from build123d import *

# Parameters (mm, degrees)
F0_W     = 70
F0_H     = 48
F0_R     = 1.6
F0_H_2   = 10
F1_DEPTH = 3.5
F2_R     = 5
F3_R     = 1


with BuildPart() as f1:
    # F0 (on Front) → F1 (new body)
    with BuildSketch(Plane.XZ):
        with Locations((18, 29)):
            Rectangle(F0_W, F0_H)
        with Locations((-11.999999, 12)):
            Circle(F0_R, mode=Mode.SUBTRACT)
        with Locations((0, 12)):
            Circle(F0_R, mode=Mode.SUBTRACT)
        with Locations((12, 12)):
            Circle(F0_R, mode=Mode.SUBTRACT)
        with Locations((24.000001, 12)):
            Circle(F0_R, mode=Mode.SUBTRACT)
        with Locations((36, 12)):
            Circle(F0_R, mode=Mode.SUBTRACT)
        with Locations((48, 12)):
            Circle(F0_R, mode=Mode.SUBTRACT)
        with Locations((-11.999999, 24)):
            Circle(F0_R, mode=Mode.SUBTRACT)
        with Locations((0, 24)):
            Circle(F0_R, mode=Mode.SUBTRACT)
        with Locations((-11.999999, 36)):
            Circle(F0_R, mode=Mode.SUBTRACT)
        with Locations((0, 36)):
            Circle(F0_R, mode=Mode.SUBTRACT)
        with Locations((12, 24)):
            Circle(F0_R, mode=Mode.SUBTRACT)
        with Locations((12, 36)):
            Circle(F0_R, mode=Mode.SUBTRACT)
        with Locations((-11.999999, 48)):
            Circle(F0_R, mode=Mode.SUBTRACT)
        with Locations((0, 48)):
            Circle(F0_R, mode=Mode.SUBTRACT)
        with Locations((12, 48)):
            Circle(F0_R, mode=Mode.SUBTRACT)
        with Locations((24.000001, 24)):
            Circle(F0_R, mode=Mode.SUBTRACT)
        with Locations((24.000001, 36)):
            Circle(F0_R, mode=Mode.SUBTRACT)
        with Locations((36, 24)):
            Circle(F0_R, mode=Mode.SUBTRACT)
        with Locations((48, 24)):
            Circle(F0_R, mode=Mode.SUBTRACT)
        with Locations((36, 36)):
            Circle(F0_R, mode=Mode.SUBTRACT)
        with Locations((48, 36)):
            Circle(F0_R, mode=Mode.SUBTRACT)
        with Locations((24.000001, 48)):
            Circle(F0_R, mode=Mode.SUBTRACT)
        with Locations((36, 48)):
            Circle(F0_R, mode=Mode.SUBTRACT)
        with Locations((48, 48)):
            Circle(F0_R, mode=Mode.SUBTRACT)
        with Locations((18, 0)):
            Rectangle(F0_W, F0_H_2)
        with Locations((-11.999999, 0)):
            Circle(F0_R, mode=Mode.SUBTRACT)
        with Locations((0, 0)):
            Circle(F0_R, mode=Mode.SUBTRACT)
        with Locations((12, 0)):
            Circle(F0_R, mode=Mode.SUBTRACT)
        with Locations((24.000001, 0)):
            Circle(F0_R, mode=Mode.SUBTRACT)
        with Locations((36, 0)):
            Circle(F0_R, mode=Mode.SUBTRACT)
        with Locations((48, 0)):
            Circle(F0_R, mode=Mode.SUBTRACT)
    extrude(amount=F1_DEPTH)

    # F2
    f2_edges = [f1.edges().sort_by_distance(p)[0] for p in [
        (-17, -1.75, -5),
        (53, -1.75, -5),
        (-17, -1.75, 53),
        (53, -1.75, 53),
    ]]
    fillet(f2_edges, radius=F2_R)

    # F3
    f3_edges = [f1.edges().sort_by_distance(p)[0] for p in [
        (18, -3.5, 53),
    ]]
    fillet(f3_edges, radius=F3_R)


solid = f1.part
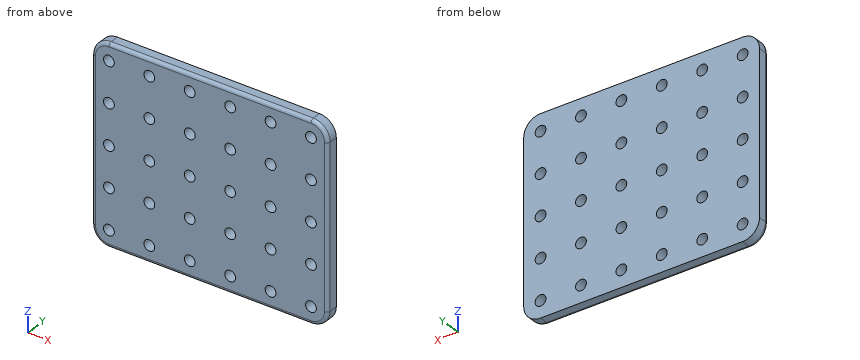
Design review of the part built by this model. Coordinates are the model's own, in mm. Give positions to 0.01 mm unless a question says otherwise; leave off trailing zeros. Loops run counter-clockwise (first coordinate to the right, second up) from the corner with the lowest first, then second, coordinate; pieces in that order, holes last. Notation, with made-up numbers: M 16.5,25.25 L 42.5,25.25 A6 cw 42.5,31.25 Z; hole C 66,19.25 d7. An arc over 180 degrees is marked long. Write item = value, one per line.
Q1. We need section A-A (z = 12). Count the separate pieces of the cut face and the enclosed holes in it, plus the area to 3 significant figures.
Output values:
separate_pieces = 7
enclosed_holes = 0
area = 177 mm^2
Q2. To check wall thickness, follow line 1 (Z direction, x = -12, y = -2.65); line 2 (Z direction, x = 47, y = -0.4); line 3 (Z direction, x = 27, y = -2.6). State the ranges of each line that lie inside material, in increasing order. Write a range as [from, to].
Output values:
line_1 = [-4.99, -1.6], [1.6, 10.4], [13.6, 22.4], [25.6, 34.4], [37.6, 46.4], [49.6, 52.99]
line_2 = [-5, -1.25], [1.25, 10.75], [13.25, 22.75], [25.25, 34.75], [37.25, 46.75], [49.25, 53]
line_3 = [-4.99, 52.99]
Q3. We need section B-B (x = 36). Give the boundary of the cut face in (y, z), plus the area to 3 significant figures.
Output values:
outline = M -3.5,-4 A1 ccw -2.5,-5 L 0,-5 L 0,-1.6 L -3.5,-1.6 Z; M -3.5,1.6 L 0,1.6 L 0,10.4 L -3.5,10.4 Z; M -3.5,13.6 L 0,13.6 L 0,22.4 L -3.5,22.4 Z; M -3.5,25.6 L 0,25.6 L 0,34.4 L -3.5,34.4 Z; M -3.5,37.6 L 0,37.6 L 0,46.4 L -3.5,46.4 Z; M -3.5,49.6 L 0,49.6 L 0,53 L -2.5,53 A1 ccw -3.5,52 Z
area = 147 mm^2
